Could you check a few things on this drawing? It's one solid part, dimensions in mm from its lowest x, y, z. Give positions to 0.01 mm unless a question says otherwise; leave off trailing zeros. Order: outer loops, then holes, each group sorted by start corner. A loop starts at its lowest first (then second) coordinate and runs counter-clockwise, first axis right, second up.
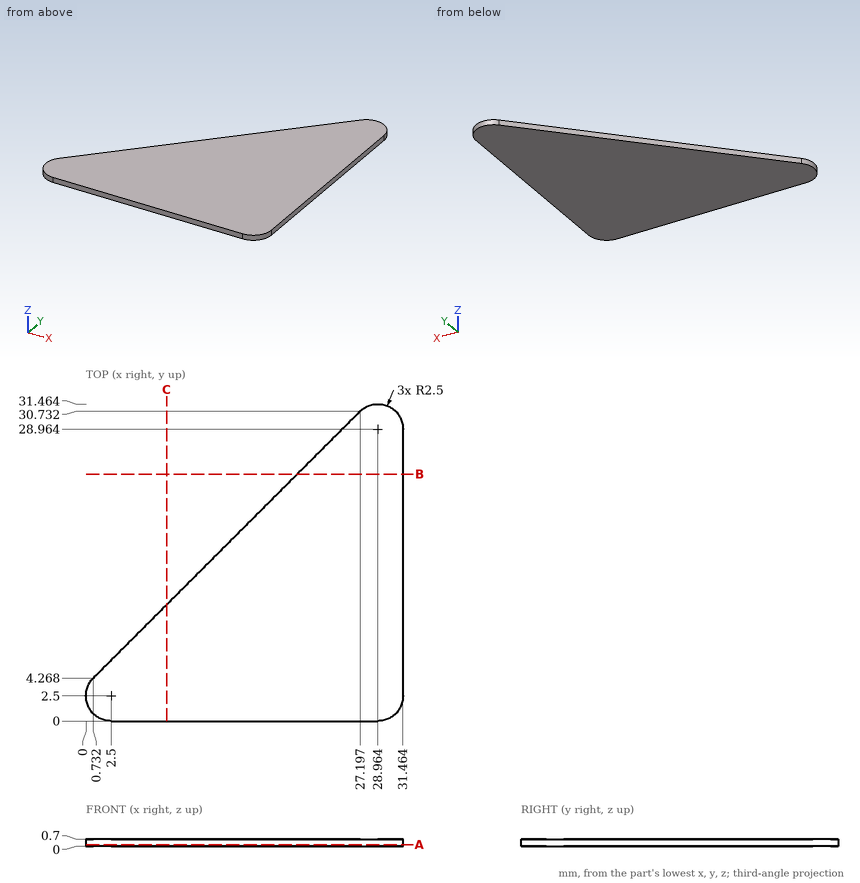
Q1. I'm going to push a flat-ended pin straight in: P1, Ø8, axis at x = 27, y = 19.5, coming from the -Z side. Where does the tip first touch, or does it pass through?
Filled sheet:
P1: stops at z = 0
Q2. If we section it at B-B on y = 24.5: List the corners of the cut face in (x, z) for me (1 decimal).
Filled sheet:
outline: (21, 0) - (31.5, 0) - (31.5, 0.7) - (21, 0.7) - close
Q3. I need wall thicknesses on L1, parallel to X at y = 20.5, z = 0.4 (1 decimal); L2, parallel to Y at x = 5, z = 0.1 (1 decimal); L3, parallel to X at y = 27, z = 0.3 (1 decimal). Which ranges of each line are inside material? Lowest first, please.
Filled sheet:
L1: x = 17 to 31.5
L2: y = 0 to 8.5
L3: x = 23.5 to 31.5
Q4. If we section it at C-C on x = 8: List the corners of the cut face in (y, z) for me (1 decimal).
Filled sheet:
outline: (0, 0) - (11.5, 0) - (11.5, 0.7) - (0, 0.7) - close
Q5. If we section it at A-A on z = 0.15: List the corners of the cut face in (x, y) for me (1 decimal).
Filled sheet:
outline: (0.7, 4.3) arc R2.5 ccw to (2.5, 0) - (29, 0) arc R2.5 ccw to (31.5, 2.5) - (31.5, 29) arc R2.5 ccw to (27.2, 30.7) - close
